```python
from build123d import *
from build123d.topology import SkipClean

# Parameters (mm, degrees)
SKETCH1_R           = 12.5
BOSS_EXTRUDE1_DEPTH = 5
SKETCH2_W           = 3
SKETCH2_H           = 12.5
SKETCH5_R           = 1.45
CUT_EXTRUDE1_DEPTH  = 5
SKETCH6_R           = 1.45
CUT_EXTRUDE2_DEPTH  = 5


with BuildPart() as part:
    # Sketch1 → Boss-Extrude1 (new, symmetric)
    with BuildSketch(Plane.XY):
        Circle(SKETCH1_R)
    extrude(amount=BOSS_EXTRUDE1_DEPTH, both=True)

    # Sketch2 → Revolve1 (revolve)
    with SkipClean():  # the faces are left unmerged after this step: merging them gives an invalid solid
        with BuildSketch(Plane(origin=(0, 0, 0), x_dir=(0, 0, -1), z_dir=(1, 0, 0)), mode=Mode.PRIVATE) as revolve1_sk:
            with Locations((-6.5, 6.25)):
                Rectangle(SKETCH2_W, SKETCH2_H)
        revolve(revolve1_sk.sketch.rotate(Axis((0, 0, 0), (0, 0, 1)), 90), axis=Axis((0, 0, 0), (0, 0, 1)))

    # Sketch5 → Cut-Extrude1 (cut)
    with SkipClean():  # the faces are left unmerged after this step: merging them gives an invalid solid
        with BuildSketch(Plane.XY.offset(8)):
            with Locations((0, 9.315)):
                Circle(SKETCH5_R)
            with Locations((9.315, 0)):
                Circle(SKETCH5_R)
            with Locations((0, -9.315)):
                Circle(SKETCH5_R)
            with Locations((-9.315, 0)):
                Circle(SKETCH5_R)
        extrude(amount=-CUT_EXTRUDE1_DEPTH, mode=Mode.SUBTRACT)

    # Sketch6 → Cut-Extrude2 (cut)
    with SkipClean():  # the faces are left unmerged after this step: merging them gives an invalid solid
        with BuildSketch(Plane(origin=(0, 0, -5), x_dir=(-1, 0, 0), z_dir=(0, 0, -1))):
            with Locations((0, 8)):
                Circle(SKETCH6_R)
            with Locations((8, 0)):
                Circle(SKETCH6_R)
            with Locations((0, -8)):
                Circle(SKETCH6_R)
            with Locations((-8, 0)):
                Circle(SKETCH6_R)
        extrude(amount=-CUT_EXTRUDE2_DEPTH, mode=Mode.SUBTRACT)


solid = part.part
```
Read the model definition and answer for the solid it produces. Units are mm, in the model's axes. A direction names the side the tool comes from. Coordinates: 2 decimals unless noted, no trailing zeros. Loops run counter-clockwise (first coordinate to the right, second up) from the corner with the lowest first, then second, coordinate; pieces in that order, holes last. Notation, with made-up numbers: (-40, 26) - (-9, 26) arc R9 ccw to (-9, 31) - close; hole circle Ø5 at (15, 33). An arc over 180 degrees is marked (long way). Answer in a Markdown table with one row per item.
1. Given pin 1 (2.5 mm diameter, centred on x = -8, y = 0, fed in from -Z); pin 2 (1 mm diameter, centred on x = 8, z = 6.5, fed in from -Y); pin 3 (2.5 mm diameter, centred on x = 9, y = 0, fed in from +Z); pin 4 (2 mm diameter, centred on y = -8.5, z = 5, fed in from -X), each flat-ended and moving along its own axis, determine where each tip first touches the part or whether it passes through.
Conclusion:
| item | result |
|---|---|
| pin 1 | stops at z = 0 |
| pin 2 | stops at y = -10 |
| pin 3 | stops at z = 8 |
| pin 4 | stops at x = -10 |
2. Find section A-A, the plane x = 0. Write down the section's boundary in (y, z) (3 decimals), then the cut area to 3 significant figures.
Conclusion:
| item | result |
|---|---|
| outline | (-12.5, -5) - (-9.45, -5) - (-9.45, 0) - (-6.55, 0) - (-6.55, -5) - (6.55, -5) - (6.55, 0) - (9.45, 0) - (9.45, -5) - (12.5, -5) - (12.5, 8) - (10.765, 8) - (10.765, 3) - (7.865, 3) - (7.865, 8) - (-7.865, 8) - (-7.865, 3) - (-10.765, 3) - (-10.765, 8) - (-12.5, 8) - close |
| area | 267 mm² |
3. Which of the six approach directions +Z, -Z, +X, -X, +Y, -Y give full straight-line access (tool end or side, diameter ignored) to faces 1 (the face through (0, 0, 8)), 2 (the face through (0, 8, 0)), 3 (the face through (-0.31, 7.9, 5.54))?
Conclusion:
| item | result |
|---|---|
| face 1 | +Z, +X, -X, +Y, -Y |
| face 2 | -Z |
| face 3 | +Z |
4. Straight lines are drawn through the part: line 1 (Y direction, x = 0, z = -1.4); line 2 (Y direction, x = 0, z = 6) (3 decimals); line 3 (X direction, y = -0.5, z = -0.25). For each, find the intervals that lie inside material, in ascending order.
Conclusion:
| item | result |
|---|---|
| line 1 | y = -12.5 to -9.45, -6.55 to 6.55, 9.45 to 12.5 |
| line 2 | y = -12.5 to -10.765, -7.865 to 7.865, 10.765 to 12.5 |
| line 3 | x = -12.49 to -9.36, -6.64 to 6.64, 9.36 to 12.49 |
5. Find section D-D, the plane y = -9. Write down the section's boundary in (x, z), then the cut area to 3 significant figures.
Conclusion:
| item | result |
|---|---|
| outline | (-8.67, -5) - (-1.05, -5) - (-1.05, 0) - (1.05, 0) - (1.05, -5) - (8.67, -5) - (8.67, 8) - (1.42, 8) - (1.42, 3) - (-1.42, 3) - (-1.42, 8) - (-8.67, 8) - close |
| area | 201 mm² |
6. Find section C-C, the plane z = 5.5. Write down the section's boundary in (x, y) (3 decimals), then the cut area to 3 significant figures.
Conclusion:
| item | result |
|---|---|
| outline | circle Ø25 at (0, 0); hole circle Ø2.9 at (-9.315, 0); hole circle Ø2.9 at (0, -9.315); hole circle Ø2.9 at (0, 9.315); hole circle Ø2.9 at (9.315, 0) |
| area | 464 mm² |
7. Determine the mould class of faces 4 (the face through (0, 0, -5)), 5 (the face through (0.314, -9.416, -2.535)) for opening direction X: +X half, -X half, draft (parallel to the pull), parting line (faces both ways), or undercut.
Conclusion:
| item | result |
|---|---|
| face 4 | draft |
| face 5 | undercut |
